Here's how the part is built. I have some questions about the finished solid (model axes, mm). Face numbers are marked on the shaded views. A direction names the side the tool comes from. Round coordinates to 2 decimals unless told otherwise and drop trailing zeros. Write each loop counter-clockwise with the first axis right and the second up, starting at its lowest first coordinate (ties: lowest second). Pieces come first, ordered by that corner, then holes. Notation, with made-up numbers: (19, 24) -> (36, 24) arc R26 cw to (36, 45) -> close; hole circle Ø7 at (80.25, -39). An arc over 180 degrees is marked (long way). Answer as CSV lines item,"result".
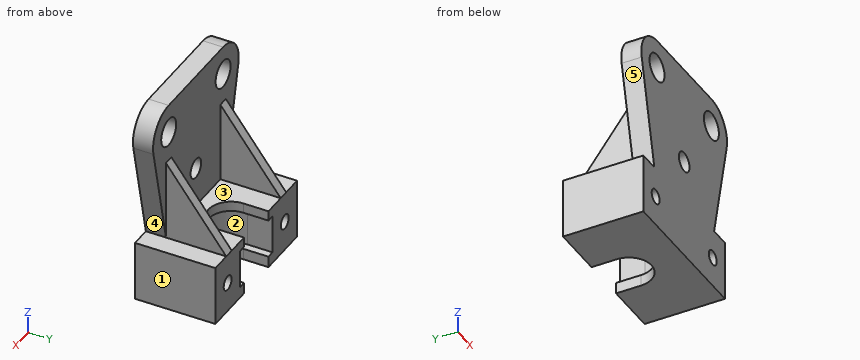
from build123d import *

# Parameters (mm, degrees)
BOSS_EXTRUDE1_DEPTH = 12
CUT_EXTRUDE1_START  = -2
CUT_EXTRUDE1_DEPTH  = 7.75
SKETCH3_R           = 1.45
CUT_EXTRUDE2_DEPTH  = 18
SKETCH4_W           = 22
SKETCH4_H           = 4
BOSS_EXTRUDE2_DEPTH = 16
SKETCH5_R           = 1.95
CUT_EXTRUDE3_DEPTH  = 14.5
BOSS_EXTRUDE3_DEPTH = 2
BOSS_EXTRUDE4_START = -22
BOSS_EXTRUDE4_DEPTH = 2
SKETCH7_R           = 2.75
BOSS_EXTRUDE5_DEPTH = 4


with BuildPart() as part:
    # Sketch1 → Boss-Extrude1 (new body)
    with BuildSketch(Plane.XY):
        with BuildLine():
            Line((-5.280588843, 25), (-5.280588843, 41))
            Line((-5.280588843, 41), (5.219411157, 41))
            Line((5.219411157, 41), (5.219411157, 36))
            ThreePointArc((5.219411157, 36), (9.719411157, 31.5), (14.219411157, 36))
            Line((14.219411157, 36), (14.219411157, 41))
            Line((14.219411157, 41), (24.719411157, 41))
            Line((24.719411157, 41), (24.719411157, 25))
            Line((24.719411157, 25), (9.719411157, 25))
            Line((9.719411157, 25), (-5.280588843, 25))
        make_face()
    extrude(amount=-BOSS_EXTRUDE1_DEPTH)

    # Sketch2 → Cut-Extrude1 (cut)
    with BuildSketch(Plane.XY.offset(CUT_EXTRUDE1_START)):
        with BuildLine():
            Line((3.719411157, 36), (3.719411157, 41))
            Line((3.719411157, 41), (15.719411157, 41))
            Line((15.719411157, 41), (15.719411157, 36))
            ThreePointArc((15.719411157, 36), (9.719411157, 30), (3.719411157, 36))
        make_face()
    extrude(amount=-CUT_EXTRUDE1_DEPTH, mode=Mode.SUBTRACT)

    # Sketch3 → Cut-Extrude2 (cut)
    with BuildSketch(Plane(origin=(0, 41, 0), x_dir=(1, 0, 0), z_dir=(0, 1, 0))):
        with Locations((20.219411157, 6)):
            Circle(SKETCH3_R)
        with Locations((-0.780588843, 6)):
            Circle(SKETCH3_R)
    extrude(amount=-CUT_EXTRUDE2_DEPTH, mode=Mode.SUBTRACT)

    # Sketch4 → Boss-Extrude2 (add)
    with BuildSketch(Plane.XY):
        with Locations((9.719411157, 27)):
            Rectangle(SKETCH4_W, SKETCH4_H)
    extrude(amount=BOSS_EXTRUDE2_DEPTH)

    # Sketch5 → Cut-Extrude3 (cut, symmetric)
    with BuildSketch(Plane(origin=(0, 29, 0), x_dir=(1, 0, 0), z_dir=(0, 1, 0))):
        with Locations((9.719411157, -8)):
            Circle(SKETCH5_R)
    extrude(amount=CUT_EXTRUDE3_DEPTH, both=True, mode=Mode.SUBTRACT)

    # Sketch6 → Boss-Extrude3 (add)
    with BuildSketch(Plane.ZY.offset(1.280588843)):
        Polygon((16, 29), (0, 41), (0, 29), align=None)
    extrude(amount=-BOSS_EXTRUDE3_DEPTH)

    # Sketch6<2> → Boss-Extrude4 (add)
    with BuildSketch(Plane.ZY.offset(1.280588843).offset(BOSS_EXTRUDE4_START)):
        Polygon((16, 29), (0, 41), (0, 29), align=None)
    extrude(amount=BOSS_EXTRUDE4_DEPTH)

    # Sketch7 → Boss-Extrude5 (add)
    with BuildSketch(Plane(origin=(0, 25, 0), x_dir=(-1, 0, 0), z_dir=(0, -1, 0))):
        with BuildLine():
            Line((1.280588843, 0), (5.893585637, -20.752295309))
            ThreePointArc((5.893585637, -20.752295309), (4.765942897, -25.597790852), (0.280588843, -27.75))
            Line((0.280588843, -27.75), (-19.719411157, -27.75))
            ThreePointArc((-19.719411157, -27.75), (-24.204765211, -25.597790852), (-25.33240795, -20.752295309))
            Line((-25.33240795, -20.752295309), (-20.719411157, 0))
            Line((-20.719411157, 0), (-20.719411157, -16))
            Line((-20.719411157, -16), (1.280588843, -16))
            Line((1.280588843, -16), (1.280588843, 0))
        make_face()
        with Locations((0.280588843, -22)):
            Circle(SKETCH7_R, mode=Mode.SUBTRACT)
        with Locations((-19.719411157, -22)):
            Circle(SKETCH7_R, mode=Mode.SUBTRACT)
    extrude(amount=-BOSS_EXTRUDE5_DEPTH)


solid = part.part
Item 1: For the marked faces 1, 2, 3, 4 and 5, which set-ups out of +Z, -Z, +X, -X, +Y, -Y let a thin tool reach every point of the face, with its end or its side?
Results found:
face 1,"-Z, +X, +Y, -Y"
face 2,"+Y"
face 3,"+Z, +Y"
face 4,"+X, +Y, -Y"
face 5,"-X, +Y, -Y"
Item 2: Suppose I cut it at C-C, the plane z = 9. List the corners of the cut face in (x, y) for me.
Results found:
outline,"(-3.28, 25) -> (8.05, 25) -> (8.05, 29) -> (0.72, 29) -> (0.72, 34.25) -> (-1.28, 34.25) -> (-1.28, 29) -> (-3.28, 29) -> close; (11.39, 25) -> (22.72, 25) -> (22.72, 29) -> (20.72, 29) -> (20.72, 34.25) -> (18.72, 34.25) -> (18.72, 29) -> (11.39, 29) -> close"
Item 3: Suppose I cut it at B-B, the plane y = 32.25. List the corners of the cut face in (x, z) for me, then the cut area to 3 significant figures.
Results found:
outline,"(-5.28, -12) -> (7.23, -12) -> (7.23, -9.75) -> (5.04, -9.75) -> (5.04, -2) -> (7.23, -2) -> (7.23, 0) -> (0.72, 0) -> (0.72, 11.67) -> (-1.28, 11.67) -> (-1.28, 0) -> (-5.28, 0) -> close; (12.21, -12) -> (24.72, -12) -> (24.72, 0) -> (20.72, 0) -> (20.72, 11.67) -> (18.72, 11.67) -> (18.72, 0) -> (12.21, 0) -> (12.21, -2) -> (14.4, -2) -> (14.4, -9.75) -> (12.21, -9.75) -> close; hole circle Ø2.9 at (-0.78, -6); hole circle Ø2.9 at (20.22, -6)"
area,"300 mm²"
Item 4: Suppose I cut it at D-D, the plane x = 15. List the corners of the cut face in (y, z) for me, then the cut area to 3 significant figures.
Results found:
outline,"(25, -12) -> (41, -12) -> (41, -9.75) -> (33.15, -9.75) -> (33.15, -2) -> (41, -2) -> (41, 0) -> (29, 0) -> (29, 27.75) -> (25, 27.75) -> close"
area,"242 mm²"
Item 5: Will these pins go through, and if not, where does the flat tip stop? pin 1 (2.5 mm diameter, centred on y = 38.5, z = -11, fed in from -X); pin 2 (2.5 mm diameter, centred on x = 9.72, z = 8, fed in from -Y); pin 3 (0.7 mm diameter, centred on y = 37.5, z = -11.5, fed in from +X); pin 4 (1.5 mm diameter, centred on x = 11, z = 20.5, fed in from +Y).
Results found:
pin 1,"stops at x = -5.28"
pin 2,"passes through"
pin 3,"stops at x = 24.72"
pin 4,"stops at y = 29"
Item 6: Suppose I cut it at A-A, the plane z = 22. List the corners of the cut face in (x, y) for me, then the cut area to 3 significant figures.
Results found:
outline,"(-6.03, 25) -> (-3.03, 25) -> (-3.03, 29) -> (-6.03, 29) -> close; (2.47, 25) -> (16.97, 25) -> (16.97, 29) -> (2.47, 29) -> close; (22.47, 25) -> (25.47, 25) -> (25.47, 29) -> (22.47, 29) -> close"
area,"82.0 mm²"
Item 7: I need wall thicknesses on L1, parallel to X at y = 29, z = -6; L2, parallel to X at y = 37.5, z = -6; L3, parallel to X at y = 27.4, z = 22. Which ranges of each line are inside material? Lowest first, please.
Results found:
L1,"x = -5.28 to -2.23, 0.67 to 18.77, 21.67 to 24.72"
L2,"x = -5.28 to -2.23, 0.67 to 3.72, 15.72 to 18.77, 21.67 to 24.72"
L3,"x = -6.03 to -3.03, 2.47 to 16.97, 22.47 to 25.47"
